from build123d import *

# Parameters (mm, degrees)
SKETCH2_R          = 1.27
CUT_EXTRUDE1_DEPTH = 12.7
SKETCH3_R          = 2
CUT_EXTRUDE2_DEPTH = 18.37099882


with BuildPart() as part:
    # Sketch1 → Revolve1 (revolve)
    with BuildSketch(Plane.XY, mode=Mode.PRIVATE) as revolve1_sk:
        Polygon((-7.5, 0), (-8.5, 0), (-8.5, -2.54), (0, -2.54), (0, 10), (-7.5, 10), align=None)
    revolve(revolve1_sk.sketch.rotate(Axis((0, 10, 0), (0, -1, 0)), 270), axis=Axis((0, 10, 0), (0, -1, 0)))

    # Sketch2 → Cut-Extrude1 (cut)
    with BuildSketch(Plane(origin=(0, 10, 0), x_dir=(1, 0, 0), z_dir=(0, 1, 0))):
        with Locations(Location((-5.55625, 0, 0), (0, 0, 270))):
            Circle(SKETCH2_R)
        with Locations(Location((5.55625, 0, 0), (0, 0, 270))):
            Circle(SKETCH2_R)
    extrude(amount=-CUT_EXTRUDE1_DEPTH, mode=Mode.SUBTRACT)

    # Sketch3 → Cut-Extrude2 (cut, through all)
    with BuildSketch(Plane.XZ.offset(2.54)):
        with Locations(Location((0, 0, 0), (0, 0, 270))):
            Circle(SKETCH3_R)
    extrude(amount=-CUT_EXTRUDE2_DEPTH, mode=Mode.SUBTRACT)


solid = part.part
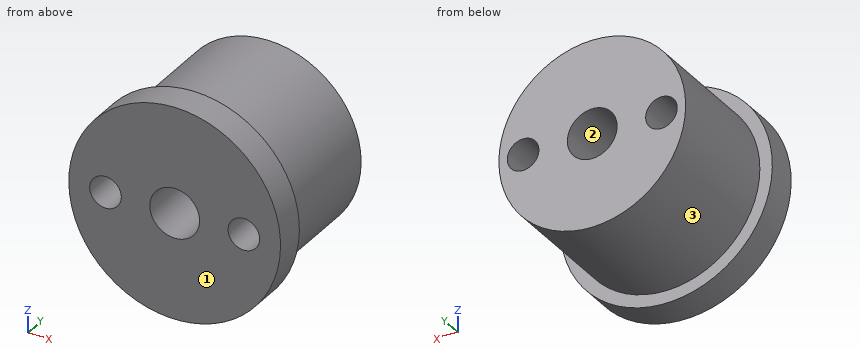
Check sheet for the modelled part. Datum: model origin and axes. Units: mm. Face numbers are marked on the shaded views. Give positions to 0.01 mm unless a question says otherwise; leave off trailing zeros. Loops run counter-clockwise (first coordinate to the right, second up) from the corner with the lowest first, then second, coordinate; pieces in that order, holes last. Notation, with made-up numbers: M 4,-40 L 16,-40 A36 ccw 16,-1 Z; hole C -26.5,73 d1. An arc over 180 degrees is marked long. Answer as a JSON object with one key per item and string values. Group by question number.
Q1. Go/stop test with flat-tipped pins: P1, Ø1.5, axis at y = 3, z = -4, coming from the +X side; P2, Ø1.5, axis at x = -5.56, z = 0, coming from the -Y side; P3, Ø5, axis at y = 8, z = 0.5, coming from the +X side; P4, Ø6, axis at y = 0.5, z = 6, coming from the -X side. Record where each tip stops, or that it passes through.
Q2. Cross-section at D-D on y = 6. Record the cut outline in (x, z).
Q3. Cross-section at A-A on x = 0. Record the cut outline in (y, z), then the cut area to 3 significant figures.
Q4. Cross-section at B-B on z = 0. Record the cut outline in (x, y).
Q5. Release check for a two-part mould opening along Z. For the marked faces 1, 2 and 3 record: released by +Z, released by -Z, zero draft, split by the parting line, or undercut.
Q6. Cross-section at C-C on x = -5.25. Record the cut outline in (y, z), then the cut area to 3 significant figures.
Q7. Material ranges on line 1 along X through (y, z) = (4.75, 0); line 2 along Y through (x, z) = (7, -4); line 3 along X through (y, z) = (-2, 7.25), recorded low to high. Write a range as [from, to].
Evaluation:
{
 "1": {"P1": "stops at x = 6.76", "P2": "passes through", "P3": "stops at x = 7.5", "P4": "stops at x = -7.94"},
 "2": {"outline": "C 0,0 d15; hole C -5.56,0 d2.54; hole C 0,0 d4; hole C 5.56,0 d2.54"},
 "3": {"outline": "M -2.54,-8.5 L 0,-8.5 L 0,-7.5 L 10,-7.5 L 10,-2 L -2.54,-2 Z; M -2.54,2 L 10,2 L 10,7.5 L 0,7.5 L 0,8.5 L -2.54,8.5 Z", "area": "143 mm2"},
 "4": {"outline": "M -8.5,-2.54 L -6.83,-2.54 L -6.83,10 L -7.5,10 L -7.5,0 L -8.5,0 Z; M -4.29,-2.54 L -2,-2.54 L -2,10 L -4.29,10 Z; M 2,-2.54 L 4.29,-2.54 L 4.29,10 L 2,10 Z; M 6.83,-2.54 L 8.5,-2.54 L 8.5,0 L 7.5,0 L 7.5,10 L 6.83,10 Z"},
 "5": {"face 1": "zero draft", "face 2": "undercut", "face 3": "split by the parting line"},
 "6": {"outline": "M -2.54,-6.68 L 0,-6.68 L 0,-5.36 L 10,-5.36 L 10,-1.23 L -2.54,-1.23 Z; M -2.54,1.23 L 10,1.23 L 10,5.36 L 0,5.36 L 0,6.68 L -2.54,6.68 Z", "area": "110 mm2"},
 "7": {"line 1": "x = [-7.5, -6.83], [-4.29, -2], [2, 4.29], [6.83, 7.5]", "line 2": "y = [-2.54, 0]", "line 3": "x = [-4.44, 4.44]"}
}
